Here's how the part is built. I have some questions about the finished solid (model axes, mm). Face numbers are marked on the shaded views. A direction names the side the tool comes from. Give positions to 0.01 mm unless a question says otherwise; leave off trailing zeros. Order: outer loops, then holes, each group sorted by start corner. A loop starts at its lowest first (then second) coordinate and runs counter-clockwise, first axis right, second up. Notation, with made-up numbers: (-14, -8.5) - (42, -8.5) arc R29 ccw to (42, 29.5) - close; hole circle Ø11 at (61, -39.5). An arc over 180 degrees is marked (long way). One line per question, with ' | ' between items.
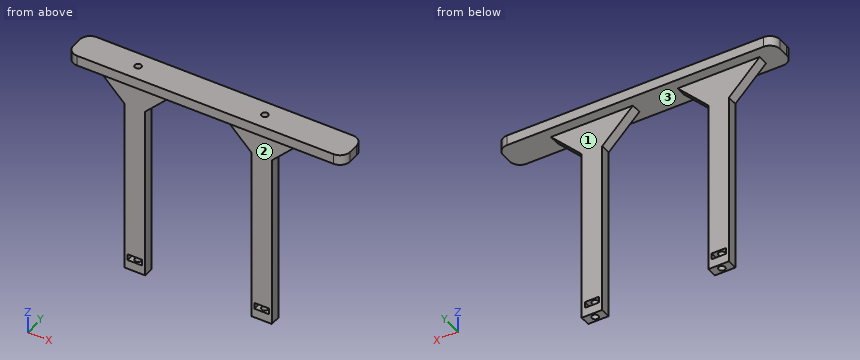
from build123d import *

# Parameters (mm, degrees)
ESBO_O1_W                  = 135
ESBO_O1_H                  = 15
RESSALTO_EXTRUS_O1_DEPTH   = 5
FILETE1_R                  = 5
FILETE2_R                  = 5
ESBO_O3_R                  = 1.6
CORTE_EXTRUS_O1_DEPTH      = 5
ESBO_O5_W                  = 10
ESBO_O5_H                  = 5
RESSALTO_EXTRUS_O4_DEPTH   = 100
RESSALTO_EXTRUS_O5_START   = -2.5
RESSALTO_EXTRUS_O5_DEPTH   = 5
RESSALTO_EXTRUS_O6_DEPTH   = 5
RESSALTO_EXTRUS_O7_START   = -2.5
RESSALTO_EXTRUS_O7_DEPTH   = 5
CORTE_EXTRUS_O2_DEPTH      = 100
CORTE_EXTRUS_O2_DEPTH_BACK = 100
ESBO_O10_W                 = 7
ESBO_O10_H                 = 3
ESBO_O11_R                 = 1.6
CORTE_EXTRUS_O3_DEPTH      = 131.673419179


with BuildPart() as part:
    # Esboço1 → Ressalto-extrusão1 (new body)
    with BuildSketch(Plane.XY):
        with Locations((9.734129461, 1.742928443)):
            Rectangle(ESBO_O1_W, ESBO_O1_H)
    extrude(amount=RESSALTO_EXTRUS_O1_DEPTH)

    # Filete1
    filete1_edges = [part.edges().sort_by_distance(p)[0] for p in [
        (-57.765870539, 9.242928443, 2.5),
        (-57.765870539, -5.757071557, 2.5),
    ]]
    fillet(filete1_edges, radius=FILETE1_R)

    # Filete2
    filete2_edges = [part.edges().sort_by_distance(p)[0] for p in [
        (77.234129461, 9.242928443, 2.5),
        (77.234129461, -5.757071557, 2.5),
    ]]
    fillet(filete2_edges, radius=FILETE2_R)

    # Esboço3 → Corte-extrusão1 (cut)
    with BuildSketch(Plane(origin=(0, 0, 0), x_dir=(-1, 0, 0), z_dir=(0, 0, -1))):
        with Locations((27.765870539, 1.742928443)):
            Circle(ESBO_O3_R)
        with Locations((-34.034129461, 1.742928443)):
            Circle(ESBO_O3_R)
    extrude(amount=-CORTE_EXTRUS_O1_DEPTH, mode=Mode.SUBTRACT)

    # Esboço5 → Ressalto-extrusão4 (add)
    with BuildSketch(Plane(origin=(0, 0, 0), x_dir=(-1, 0, 0), z_dir=(0, 0, -1))):
        with Locations((-34.034129461, 1.742928443)):
            Rectangle(ESBO_O5_W, ESBO_O5_H)
        with Locations((27.765870539, 1.742928443)):
            Rectangle(ESBO_O5_W, ESBO_O5_H)
    extrude(amount=RESSALTO_EXTRUS_O4_DEPTH)

    # Esboço7 → Ressalto-extrusão5 (add)
    with BuildSketch(Plane(origin=(0, 1.742928443, 0), x_dir=(1, 0, 0), z_dir=(0, 1, 0)).offset(RESSALTO_EXTRUS_O5_START)):
        Polygon((-32.765870539, 15), (-32.765870539, 0), (-47.765870539, 0), align=None)
    extrude(amount=RESSALTO_EXTRUS_O5_DEPTH)

    # Esboço8 → Ressalto-extrusão6 (add)
    with BuildSketch(Plane(origin=(0, 4.242928443, 0), x_dir=(1, 0, 0), z_dir=(0, 1, 0))):
        Polygon((39.034129461, 15), (39.034129461, 0), (54.034129461, 0), align=None)
    extrude(amount=-RESSALTO_EXTRUS_O6_DEPTH)

    # Esboço9 → Ressalto-extrusão7 (add)
    with BuildSketch(Plane(origin=(0, 1.742928443, 0), x_dir=(1, 0, 0), z_dir=(0, 1, 0)).offset(RESSALTO_EXTRUS_O7_START)):
        Polygon((29.034129461, 0), (14.034129461, 0), (29.034129461, 15), align=None)
        Polygon((-7.765870539, 0), (-22.765870539, 0), (-22.765870539, 15), align=None)
    extrude(amount=RESSALTO_EXTRUS_O7_DEPTH)

    # Esboço10 → Corte-extrusão2 (cut, two sides: drawn at the far end of the back side and taken through both)
    with BuildSketch(Plane(origin=(0, 1.742928443, 0), x_dir=(1, 0, 0), z_dir=(0, 1, 0)).offset(-CORTE_EXTRUS_O2_DEPTH_BACK)):
        with Locations((-27.765870539, 94)):
            Rectangle(ESBO_O10_W, ESBO_O10_H)
        with Locations((34.034129461, 94)):
            Rectangle(ESBO_O10_W, ESBO_O10_H)
    extrude(amount=CORTE_EXTRUS_O2_DEPTH + CORTE_EXTRUS_O2_DEPTH_BACK, mode=Mode.SUBTRACT)

    # Esboço11 → Corte-extrusão3 (cut, through all)
    with BuildSketch(Plane(origin=(0, 0, -100), x_dir=(-1, 0, 0), z_dir=(0, 0, -1))):
        with Locations((27.765870539, 1.742928443)):
            Circle(ESBO_O11_R)
        with Locations((-34.034129461, 1.742928443)):
            Circle(ESBO_O11_R)
    extrude(amount=-CORTE_EXTRUS_O3_DEPTH, mode=Mode.SUBTRACT)


solid = part.part
1) I want a section at C-C (y = 7.75). List the corners of the cut face in (x, z) for me, plus the area to 3 significant figures.
Model answer:
outline: (-56.33, 0) - (75.8, 0) - (75.8, 5) - (-56.33, 5) - close | area: 661 mm2
2) I want a section at B-B (x = 26). List the corners of the cut face in (y, z) for me.
Model answer:
outline: (-5.76, 0) - (-0.76, 0) - (-0.76, -11.97) - (4.24, -11.97) - (4.24, 0) - (9.24, 0) - (9.24, 5) - (-5.76, 5) - close
3) Please list where these lines run through material, in increasing order: L1, parallel to X at y = 3.5, z = -78.5; L2, parallel to X at y = 1, z = -66.5; L3, parallel to X at y = 2.25, z = -54.
Model answer:
L1: x = -32.77 to -22.77, 29.03 to 39.03 | L2: x = -32.77 to -29.18, -26.35 to -22.77, 29.03 to 32.62, 35.45 to 39.03 | L3: x = -32.77 to -29.28, -26.25 to -22.77, 29.03 to 32.52, 35.55 to 39.03
4) On a 3-axis mill with a long thin cutter (end or side, diameter ignored), from which of +Z, -Z, +X, -X, +Y, -Y can I reach the whole of each face in a straight line? I mean the marked faces 1, 2 and 3. Say none if no direction works.
Model answer:
face 1: -Z, +X, -X, +Y | face 2: -Z, +X, -X, -Y | face 3: -Z
5) I'm going to push flat-ended pins straight in: P1, Ø2.5, axis at x = 34.03, y = 1.74, coming from the -Z side; P2, Ø1.5, axis at x = 35.5, y = 2, coming from the -Z side; P3, Ø2.5, axis at y = 1, z = -58, coming from the +X side; P4, Ø1.5, axis at y = 1, z = -42, coming from the -X side. Where does each tip first touch, or does it pass through?
Model answer:
P1: passes through | P2: stops at z = -100 | P3: stops at x = 39.03 | P4: stops at x = -32.77
6) I want a section at A-A (z = -61). List the corners of the cut face in (x, y) for me, plus the area to 3 significant figures.
Model answer:
outline: (-32.77, -0.76) - (-22.77, -0.76) - (-22.77, 4.24) - (-32.77, 4.24) - close; (29.03, -0.76) - (39.03, -0.76) - (39.03, 4.24) - (29.03, 4.24) - close; hole circle Ø3.2 at (-27.77, 1.74); hole circle Ø3.2 at (34.03, 1.74) | area: 83.9 mm2
7) I want a section at D-D (x = 48). List the corners of the cut face in (y, z) for me.
Model answer:
outline: (-5.76, 0) - (-0.76, 0) - (-0.76, -6.03) - (4.24, -6.03) - (4.24, 0) - (9.24, 0) - (9.24, 5) - (-5.76, 5) - close
